```python
from build123d import *

# Parameters (mm, degrees)
SKETCH2_W           = 63
SKETCH2_H           = 52
BOSS_EXTRUDE1_DEPTH = 31
SKETCH1_W           = 57
SKETCH1_H           = 46
CUT_EXTRUDE1_DEPTH  = 31
SKETCH3_W           = 3
SKETCH3_H           = 46
CUT_EXTRUDE2_DEPTH  = 5
SKETCH4_W           = 52
SKETCH4_H           = 3
BOSS_EXTRUDE2_DEPTH = 17
SKETCH5_W           = 10
SKETCH5_H           = 52
BOSS_EXTRUDE3_DEPTH = 3


with BuildPart() as part:
    # Sketch2 → Boss-Extrude1 (new body)
    with BuildSketch(Plane(origin=(0, 0, 0), x_dir=(1, 0, 0), z_dir=(0, 1, 0))):
        with Locations((28.5, -23)):
            Rectangle(SKETCH2_W, SKETCH2_H)
    extrude(amount=BOSS_EXTRUDE1_DEPTH)

    # Sketch1 → Cut-Extrude1 (cut)
    with BuildSketch(Plane(origin=(0, 0, 0), x_dir=(1, 0, 0), z_dir=(0, 1, 0))):
        with Locations((28.5, -23)):
            Rectangle(SKETCH1_W, SKETCH1_H)
    extrude(amount=CUT_EXTRUDE1_DEPTH, mode=Mode.SUBTRACT)

    # Sketch3 → Cut-Extrude2 (cut)
    with BuildSketch(Plane.XZ):
        with Locations((58.5, 23)):
            Rectangle(SKETCH3_W, SKETCH3_H)
    extrude(amount=-CUT_EXTRUDE2_DEPTH, mode=Mode.SUBTRACT)

    # Sketch4 → Boss-Extrude2 (add)
    with BuildSketch(Plane(origin=(0, 0, 46), x_dir=(-1, 0, 0), z_dir=(0, 0, -1))):
        with Locations((-26, 9.5)):
            Rectangle(SKETCH4_W, SKETCH4_H)
    extrude(amount=BOSS_EXTRUDE2_DEPTH)

    # Sketch5 → Boss-Extrude3 (add)
    with BuildSketch(Plane(origin=(0, 31, 0), x_dir=(1, 0, 0), z_dir=(0, 1, 0))):
        with Locations((2, -23)):
            Rectangle(SKETCH5_W, SKETCH5_H)
    extrude(amount=BOSS_EXTRUDE3_DEPTH)


solid = part.part
```
The listing builds one solid part. Answer for the finished solid, in the listing's coordinates (mm). A direction names the side the tool comes from. Give positions to 0.01 mm unless a question says otherwise; leave off trailing zeros. Order: outer loops, then holes, each group sorted by start corner. A loop starts at its lowest first (then second) coordinate and runs counter-clockwise, first axis right, second up. Notation, with made-up numbers: (9.25, -1) -> (53.25, -1) arc R25 ccw to (53.25, 26) -> close; hole circle Ø2 at (26.25, 40.5). An arc over 180 degrees is marked (long way). One line per item, written item: value.
1) Find the intervals of material crossed by line 1 (X direction, y = 18, z = 0.5); line 2 (Z direction, x = 10, y = 14); line 3 (Y direction, x = 6.5, z = 41), in increasing order.
Reported:
line 1: x = -3 to 0, 57 to 60
line 2: z = -3 to 0, 46 to 49
line 3: y = 8 to 11, 31 to 34
2) Determine the mould class of faces 1 (the flat face through (28, 17, 49)), 2 (the flat face through (-3, 17, 23)), 3 (the flat face through (26, 11, 38)) for opening direction Z: pulls with the +Z half, pulls with the -Z half, needs draft (parallel to the pull), parting line crosses it, or undercut.
Reported:
face 1: pulls with the +Z half
face 2: needs draft
face 3: undercut
3) Find section C-C, the plane y = 17. Determine the outline of the cut face in (x, z).
Reported:
outline: (-3, -3) -> (60, -3) -> (60, 49) -> (-3, 49) -> close; hole (0, 0) -> (57, 0) -> (57, 46) -> (0, 46) -> close
4) A tool of negligible diameter and unlimited length cuts with its end or side. For faces 4 (the flat face through (39.3, 31, -0.2)), 5 (the flat face through (3, 31, 23)), 6 (the flat face through (57, 18, 23)), 7 (the flat face through (58, 5, 23)), 8 (the flat face through (26, 8, 38)), from which of +Z, -Z, +X, -X, +Y, -Y can it reach the whole face along a straight path? Write none if from no direction.
Reported:
face 4: +Z, -Z, +X, +Y
face 5: none
face 6: +Y, -Y
face 7: +X, -Y
face 8: -Y
5) Flat-ended cylindrical pins translate along their axes: P1, Ø1.5, axis at y = 32, z = 17, coming from the +X side; P2, Ø5, axis at x = 26.5, z = 38.5, coming from the +Y side; P3, Ø7.5, axis at x = 4, z = 33, coming from the -Y side; P4, Ø4, axis at x = 10, z = 4.5, coming from the -Y side. Find the tip coordinate at first contact, or state that the pin passes through.
Reported:
P1: stops at x = 7
P2: stops at y = 11
P3: stops at y = 8
P4: passes through
6) Find section A-A, the plane x = 27.5. Determine the outline of the cut face in (y, z).
Reported:
outline: (0, -3) -> (31, -3) -> (31, 0) -> (0, 0) -> close; (0, 46) -> (8, 46) -> (8, 29) -> (11, 29) -> (11, 46) -> (31, 46) -> (31, 49) -> (0, 49) -> close
7) Find section B-B, the plane z = 33.5. Determine the outline of the cut face in (x, y), plus the area to 3 significant figures.
Reported:
outline: (-3, 0) -> (0, 0) -> (0, 8) -> (52, 8) -> (52, 11) -> (0, 11) -> (0, 31) -> (7, 31) -> (7, 34) -> (-3, 34) -> close; (57, 5) -> (60, 5) -> (60, 31) -> (57, 31) -> close
area: 357 mm^2
8) Find section D-D, the plane y = 3.5. Determine the outline of the cut face in (x, z), plus the area to 3 significant figures.
Reported:
outline: (-3, -3) -> (60, -3) -> (60, 0) -> (0, 0) -> (0, 46) -> (60, 46) -> (60, 49) -> (-3, 49) -> close
area: 516 mm^2
